The listing builds one solid part. Answer for the finished solid, in the listing's coordinates (mm). Round coordinates to 2 decimals unless told otherwise and drop trailing zeros. Order: outer loops, then holes, each group sorted by start corner. A loop starts at its lowest first (then second) coordinate and runs counter-clockwise, first axis right, second up. Notation, with made-up numbers: (23, -17) -> (64, -17) arc R10 cw to (64, -6) -> close; hole circle Ø9 at (16, -29.5). An arc over 180 degrees is marked (long way). Return JSON: item names as keys, results as strings. Group by question number.
(1) Consider line 1 (X direction, y = 13, z = 1.5); line 2 (Y direction, x = 0, z = 1.2); line 3 (Y direction, x = -6, z = 0.5). Determine where each line is inside the solid, lowest interval first. Write a range as [from, to].
(2) The part is cut by section A-A (y = 0). Determine the outline of the cut face in (x, z).
(3) The part is cut by section C-C (z = 0.3). Determine the outline of the cut face in (x, y), plus the area to 3 significant figures.
from build123d import *

# Parameters (mm, degrees)
CYLINDER009_R     = 17.5
CYLINDER009_DEPTH = 10


with BuildPart() as cylinder009:
    # Cylinder009 → Cylinder009 (new body)
    with BuildSketch(Plane.XY):
        Circle(CYLINDER009_R)
    extrude(amount=CYLINDER009_DEPTH)


with BuildPart() as cut009:
    # Cone008 → Cone008 (revolve)
    with BuildSketch(Plane.XZ):
        Polygon((0, 0), (25.5, 0), (25.7, 2), (0, 2), align=None)
    revolve(axis=Axis((0, 0, 0), (0, 0, 1)))

    # Cut009: cut Cylinder009
    add(cylinder009.part, mode=Mode.SUBTRACT)


solid = cut009.part
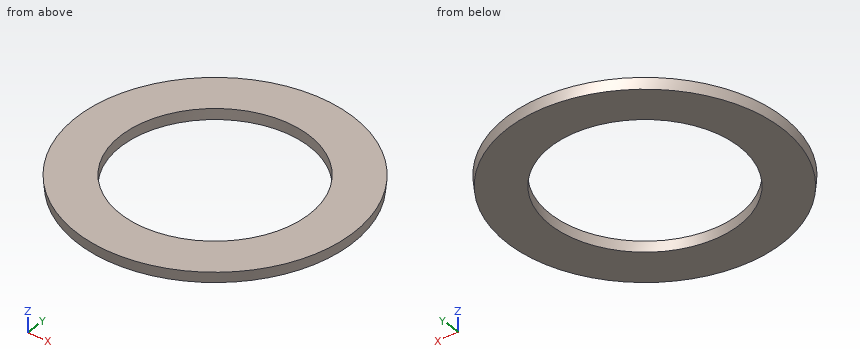
Answer below:
{
 "1": {"line 1": "x = [-22.11, -11.72], [11.72, 22.11]", "line 2": "y = [-25.62, -17.5], [17.5, 25.62]", "line 3": "y = [-24.84, -16.44], [16.44, 24.84]"},
 "2": {"outline": "(-25.7, 2) -> (-25.5, 0) -> (-17.5, 0) -> (-17.5, 2) -> close; (17.5, 0) -> (25.5, 0) -> (25.7, 2) -> (17.5, 2) -> close"},
 "3": {"outline": "circle Ø51.06 at (0, 0); hole circle Ø35 at (0, 0)", "area": "1,090 mm²"}
}
